```python
from build123d import *

# Parameters (mm, degrees)
F0_R          = 50.8
F1_DEPTH      = 25.4
F2_R          = 5.08
F3_DEPTH      = 139.7
F3_DEPTH_BACK = 139.7
F4_R          = 5.08
F5_DEPTH      = 139.7
F5_DEPTH_BACK = 139.7
F6_R          = 11.43
F7_DEPTH      = 27.94


with BuildPart() as f1:
    # F0 (on Front) → F1 (new body)
    with BuildSketch(Plane.XZ):
        Circle(F0_R)
    extrude(amount=F1_DEPTH)

    # F2 (on Right) → F3 (join, two sides)
    with BuildSketch(Plane.YZ) as f3_sk:
        with Locations((-12.7, 0)):
            Circle(F2_R)
    extrude(amount=F3_DEPTH)
    extrude(f3_sk.sketch, amount=-F3_DEPTH_BACK)

    # F4 (on Top) → F5 (join, two sides)
    with BuildSketch(Plane.XY) as f5_sk:
        with Locations((0, -12.7)):
            Circle(F4_R)
    extrude(amount=F5_DEPTH)
    extrude(f5_sk.sketch, amount=-F5_DEPTH_BACK)

    # F6 (on Front) → F7 (cut)
    with BuildSketch(Plane.XZ):
        Circle(F6_R)
    extrude(amount=F7_DEPTH, mode=Mode.SUBTRACT)


solid = f1.part
```
The listing builds one solid part. Answer for the finished solid, in the listing's coordinates (mm). A direction names the side the tool comes from. Coordinates: 2 decimals unless noted, no trailing zeros. Write each loop counter-clockwise with the first axis right and the second up, starting at its lowest first coordinate (ties: lowest second). Pieces come first, ordered by that corner, then holes. Notation, with made-up numbers: (38, -19) - (61, -19) arc R19 ccw to (61, -13) - close; hole circle Ø3 at (-6, 4.25). An arc over 180 degrees is marked (long way). Return JSON: item names as keys, results as strings. Group by question number.
1. Straight lines are drawn through the part: L1, parallel to X at y = -19.5, z = 0; L2, parallel to Z at x = 0, y = -17. For each, find the intervals that lie inside material, in ascending order.
2. A cutting plane is placed at C-C, the plane x = -83. Determine the outline of the cut face in (y, z), plus the area to 3 significant figures.
3. A cutting plane is placed at B-B, the plane z = 0. Determine the outline of the cut face in (x, y), plus the area to 3 significant figures.
4. A cutting plane is placed at D-D, the plane z = -66. Determine the outline of the cut face in (x, y).
5. Determine the mould class of faces 1 (the cylindrical face through (-1.1, -17.66, -94.5)), 2 (the cylindrical face through (10.902, -12.522, 3.433)), 3 (the cylindrical face through (94.5, -16.73, -3.09)), 4 (the flat face through (-139.7, -13, 0)) for opening direction X: released by +X, released by -X, zero draft, split by the parting line, or undercut.
6. Given pin 1 (1.5 mm diameter, centred on x = 88, z = 2.5, fed in from -Y); pin 2 (4 mm diameter, centred on y = -7.5, z = -28.5, fed in from -X); pin 3 (6 mm diameter, centred on y = -7.5, z = 105, fed in from +X); pin 4 (3 mm diameter, centred on x = 58.5, y = -19.5, fed in from +Z), each flat-ended and moving along its own axis, determine where each tip first touches the part or whether it passes through.
7. A cutting plane is placed at A-A, the plane y = -12.7. Determine the outline of the cut face in (x, z).
8. Which of the six approach directions +Z, -Z, +X, -X, +Y, -Y give full straight-line access (tool end or side, diameter ignored) to faces 5 (the cylindrical face through (-1.1, -17.66, 94.5)), 6 (the cylindrical face through (-94.5, -16.73, -3.09)), 7 (the flat face through (-1, 0, 12))?
Ans:
{
 "1": {"L1": "-50.8 to -11.43, 11.43 to 50.8", "L2": "-139.7 to -11.43, 11.43 to 139.7"},
 "2": {"outline": "circle Ø10.16 at (-12.7, 0)", "area": "81.1 mm²"},
 "3": {"outline": "(-139.7, -17.78) - (-50.8, -17.78) - (-50.8, -25.4) - (-11.43, -25.4) - (-11.43, 0) - (-50.8, 0) - (-50.8, -7.62) - (-139.7, -7.62) - close; (11.43, -25.4) - (50.8, -25.4) - (50.8, -17.78) - (139.7, -17.78) - (139.7, -7.62) - (50.8, -7.62) - (50.8, 0) - (11.43, 0) - close", "area": "3,810 mm²"},
 "4": {"outline": "circle Ø10.16 at (0, -12.7)"},
 "5": {"face 1": "split by the parting line", "face 2": "undercut", "face 3": "zero draft", "face 4": "released by -X"},
 "6": {"pin 1": "y = -17.47", "pin 2": "x = -43.34", "pin 3": "x = 4.58", "pin 4": "through"},
 "7": {"outline": "(-139.7, -5.08) - (-50.55, -5.08) arc R50.8 ccw to (-5.08, -50.55) - (-5.08, -139.7) - (5.08, -139.7) - (5.08, -50.55) arc R50.8 ccw to (50.55, -5.08) - (139.7, -5.08) - (139.7, 5.08) - (50.55, 5.08) arc R50.8 ccw to (5.08, 50.55) - (5.08, 139.7) - (-5.08, 139.7) - (-5.08, 50.55) arc R50.8 ccw to (-50.55, 5.08) - (-139.7, 5.08) - close; hole circle Ø22.86 at (0, 0)"},
 "8": {"face 5": "+Z", "face 6": "-X", "face 7": "+Z, -Z, +X, -X, +Y"}
}
